Geometry: see drawing. Coordinates: mm, zero at the bounding-box minimum. Round coordinates to 2 decimals unless told otherwise and drop trailing zeros. Write each loop counter-clockwise with the first axis right and the second up, starting at its lowest first coordinate (ties: lowest second). Pieces come first, ordered by that corner, then holes. Notation, with made-up numbers: M 74,47 L 83,47 A17 cw 83,59 Z; hole C -16.75,14.5 d3. An arc over 180 degrees is marked long. Use one line per item in the form item = value. Start each with the question number.
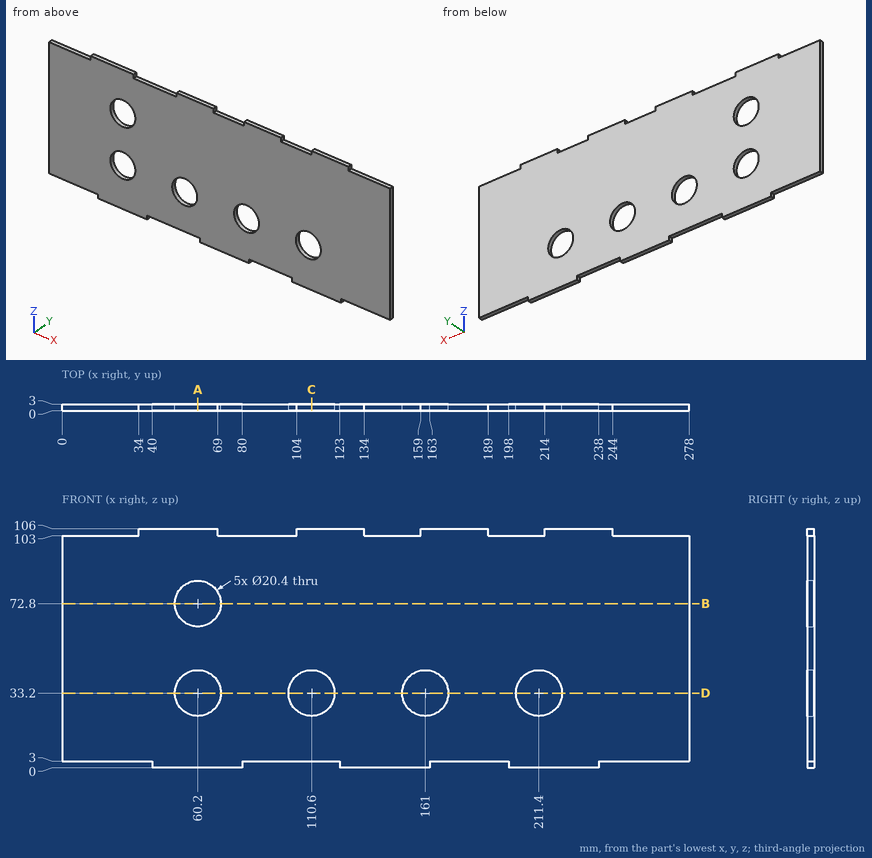
Item 1: Cut plane B-B (z = 72.8). Output: boundary loops of the cut face in (x, y), plus the area to 3 significant figures.
Item 2: Cut plane C-C (x = 110.6). Output: boundary loops of the cut face in (y, z).
Item 3: Ray query, line 1 (X direction, y = 1.8, z = 33.2); line 2 (X direction, y = 1.8, z = 72.8); line 3 (Z direction, x = 111, y = 1.15). Return the intervals inside material, ascending. Write a range as from..to.
Item 4: Cut plane A-A (x = 60.2). Output: boundary loops of the cut face in (y, z), plus the area to 3 significant figures.
Item 5: First-contact query: pin 1 (1.5 mm diameter, centred on y = 1, z = 105, fed in from +X); pin 2 (1.5 mm diameter, centred on x = 184.5, y = 2, fed in from -Z); pin 3 (0.9 mm diameter, centred on y = 1.5, z = 2, fed in from -X). Flat tips, straight axial feed; report the tip coordinate or a pass-through.
Item 6: Cut plane D-D (z = 33.2). Output: boundary loops of the cut face in (x, y), plus the area to 3 significant figures.
Final values:
q1.outline = M 0,0 L 50,0 L 50,3 L 0,3 Z; M 70.4,0 L 278,0 L 278,3 L 70.4,3 Z
q1.area = 773 mm^2
q2.outline = M 0,3 L 3,3 L 3,23 L 0,23 Z; M 0,43.4 L 3,43.4 L 3,106 L 0,106 Z
q3.line_1 = 0..50, 70.4..100.4, 120.8..150.8, 171.2..201.2, 221.6..278
q3.line_2 = 0..50, 70.4..278
q3.line_3 = 3..23.01, 43.39..106
q4.outline = M 0,0 L 3,0 L 3,23 L 0,23 Z; M 0,43.4 L 3,43.4 L 3,62.6 L 0,62.6 Z; M 0,83 L 3,83 L 3,106 L 0,106 Z
q4.area = 196 mm^2
q5.pin_1 = 244
q5.pin_2 = 3
q5.pin_3 = 40
q6.outline = M 0,0 L 50,0 L 50,3 L 0,3 Z; M 70.4,0 L 100.4,0 L 100.4,3 L 70.4,3 Z; M 120.8,0 L 150.8,0 L 150.8,3 L 120.8,3 Z; M 171.2,0 L 201.2,0 L 201.2,3 L 171.2,3 Z; M 221.6,0 L 278,0 L 278,3 L 221.6,3 Z
q6.area = 589 mm^2
